Could you check a few things on this model? Use its own coordinates, in mm. Round coordinates to 2 decimals unless told otherwise and drop trailing zeros. Loops run counter-clockwise (first coordinate to the right, second up) from the corner with the lowest first, then second, coordinate; pieces in that order, holes last.
from build123d import *

# Parameters (mm, degrees)
SKETCH_1_W           = 250
SKETCH_1_H           = 140
EXTRUDE_1_DEPTH      = 4
SKETCH_2_R           = 1.55
CUT_EXTRUDE_1_DEPTH  = 4
SKETCH_4_W           = 350
SKETCH_4_H           = 30
EXTRUDE_2_DEPTH      = 4
EXTRUDE_3_DEPTH      = 4
SKETCH_3_R           = 2.05
CUT_EXTRUDE_2_DEPTH  = 4
SKETCH_6_W           = 189.5
SKETCH_6_H           = 45
CUT_EXTRUDE_3_DEPTH  = 4
CUT_EXTRUDE_4_DEPTH  = 4
CUT_EXTRUDE_5_DEPTH  = 4
FILLET_1_R           = 10
CUT_EXTRUDE_6_DEPTH  = 4
CUT_EXTRUDE_7_DEPTH  = 4
FILLET_2_R           = 2
FILLET_3_R           = 10
FILLET_4_R           = 30
SKETCH_11_R          = 1.55
EXTRUDE_4_DEPTH      = 4
EXTRUDE_START        = -4
EXTRUDE_5_DEPTH      = 4
SKETCH_13_R          = 2.1
CUT_EXTRUDE_12_DEPTH = 4
FILLET_5_R           = 2


with BuildPart() as part:
    # 草图1 → 凸台-拉伸1 (new body)
    with BuildSketch(Plane.XY):
        Rectangle(SKETCH_1_W, SKETCH_1_H)
    extrude(amount=EXTRUDE_1_DEPTH)

    # 草图2 → 切除-拉伸1 (cut)
    with BuildSketch(Plane.XY.offset(4)):
        with Locations((-108.75, 65)):
            Circle(SKETCH_2_R)
        with Locations((-108.75, 38.2)):
            Circle(SKETCH_2_R)
        with Locations((108.75, 65)):
            Circle(SKETCH_2_R)
        with Locations((108.75, 38.2)):
            Circle(SKETCH_2_R)
    extrude(amount=-CUT_EXTRUDE_1_DEPTH, mode=Mode.SUBTRACT)

    # 草图4 → 凸台-拉伸2 (add)
    with BuildSketch(Plane.XY.offset(4)):
        with Locations((0, -55)):
            Rectangle(SKETCH_4_W, SKETCH_4_H)
    extrude(amount=-EXTRUDE_2_DEPTH)

    # 草图5 → 凸台-拉伸3 (add)
    with BuildSketch(Plane.XY.offset(4)):
        Polygon((-125, -40), (-125, 70), (-175, -40), align=None)
        Polygon((175, -40), (125, 70), (125, -40), align=None)
    extrude(amount=-EXTRUDE_3_DEPTH)

    # 草图3 → 切除-拉伸2 (cut)
    with BuildSketch(Plane.XY.offset(4)):
        with Locations((50, -56.4)):
            Circle(SKETCH_3_R)
        with Locations((0, -56.4)):
            Circle(SKETCH_3_R)
        with Locations((100, -56.4)):
            Circle(SKETCH_3_R)
        with Locations((150, -56.4)):
            Circle(SKETCH_3_R)
        with Locations((-50, -56.4)):
            Circle(SKETCH_3_R)
        with Locations((-100, -56.4)):
            Circle(SKETCH_3_R)
        with Locations((-150, -56.4)):
            Circle(SKETCH_3_R)
    extrude(amount=-CUT_EXTRUDE_2_DEPTH, mode=Mode.SUBTRACT)

    # 草图6 → 切除-拉伸3 (cut)
    with BuildSketch(Plane.XY.offset(4)):
        with Locations((0, 47.5)):
            Rectangle(SKETCH_6_W, SKETCH_6_H)
    extrude(amount=-CUT_EXTRUDE_3_DEPTH, mode=Mode.SUBTRACT)

    # 草图7 → 切除-拉伸4 (cut)
    with BuildSketch(Plane.XY.offset(4)):
        Polygon((-125, 70), (-125, 30), (-175, -40), align=None)
        Polygon((175, -40), (125, 70), (125, 30), align=None)
    extrude(amount=-CUT_EXTRUDE_4_DEPTH, mode=Mode.SUBTRACT)

    # 草图8 → 切除-拉伸5 (cut)
    with BuildSketch(Plane.XY.offset(4)):
        with BuildLine():
            Line((-150, -63.9), (150, -63.9))
            ThreePointArc((150, -63.9), (156.178018616, -60.652303609), (157.005549561, -53.721889595))
            Line((157.005549561, -53.721889595), (125, 30))
            Line((125, 30), (228.155592589, 30))
            Line((228.155592589, 30), (175, -70))
            Line((175, -70), (-175, -70))
            Line((-175, -70), (-228.155592589, 30))
            Line((-228.155592589, 30), (-125, 30))
            Line((-125, 30), (-157.005549561, -53.721889595))
            ThreePointArc((-157.005549561, -53.721889595), (-156.178018616, -60.652303609), (-150, -63.9))
        make_face()
    extrude(amount=-CUT_EXTRUDE_5_DEPTH, mode=Mode.SUBTRACT)

    # 圆角1
    fillet_1_edges = [part.edges().sort_by_distance(p)[0] for p in [
        (94.75, 25, 2),
        (-94.75, 25, 2),
    ]]
    fillet(fillet_1_edges, radius=FILLET_1_R)

    # 草图9 → 切除-拉伸6 (cut)
    with BuildSketch(Plane.XY.offset(4)):
        Polygon((-57, -39.42450978), (-57, -46.4), (-4, -46.4), (-4, -22.251950414), align=None)
        Polygon((-57, -2.487306614), (-57, -28.912693386), (-16.221410479, -15.7), align=None)
        Polygon((-57, 15), (-57, 8.02450978), (-4, -9.148049586), (-4, 15), align=None)
        Polygon((4, 15), (4, -9.148049586), (57, 8.02450978), (57, 15), align=None)
        Polygon((16.221410479, -15.7), (57, -28.912693386), (57, -2.487306614), align=None)
        Polygon((4, -22.251950414), (4, -46.4), (57, -46.4), (57, -39.42450978), align=None)
        Polygon((63, -0.54324329), (63, -30.85675671), (94.75, -41.144091803), (94.75, 9.744091803), align=None)
        Polygon((-94.75, -41.144091803), (-63, -30.85675671), (-63, -0.54324329), (-94.75, 9.744091803), align=None)
    extrude(amount=-CUT_EXTRUDE_6_DEPTH, mode=Mode.SUBTRACT)

    # 草图10 → 切除-拉伸7 (cut)
    with BuildSketch(Plane.XY.offset(4)):
        Polygon((-100.75, 28.2), (-100.75, -46.4), (-145.641868809, -46.4), (-117.123472857, 28.2), align=None)
        Polygon((117.123472857, 28.2), (100.75, 28.2), (100.75, -46.4), (145.641868809, -46.4), align=None)
    extrude(amount=-CUT_EXTRUDE_7_DEPTH, mode=Mode.SUBTRACT)

    # 圆角2
    fillet_2_edges = [part.edges().sort_by_distance(p)[0] for p in [
        (-57, 15, 2),
        (-4, 15, 2),
        (-4, -9.148049586, 2),
        (-57, 8.02450978, 2),
        (-57, -2.487306614, 2),
        (-16.221410479, -15.7, 2),
        (-57, -28.912693386, 2),
        (57, -2.487306614, 2),
        (57, -28.912693386, 2),
        (16.221410479, -15.7, 2),
        (57, 15, 2),
        (57, 8.02450978, 2),
        (4, -9.148049586, 2),
        (4, 15, 2),
        (57, -39.42450978, 2),
        (57, -46.4, 2),
        (4, -46.4, 2),
        (4, -22.251950414, 2),
        (63, -0.54324329, 2),
        (94.75, 9.744091803, 2),
        (94.75, -41.144091803, 2),
        (63, -30.85675671, 2),
        (-63, -0.54324329, 2),
        (-63, -30.85675671, 2),
        (-94.75, -41.144091803, 2),
        (-94.75, 9.744091803, 2),
        (-57, -39.42450978, 2),
        (-4, -22.251950414, 2),
        (-4, -46.4, 2),
        (-57, -46.4, 2),
        (-100.75, -46.4, 2),
        (-145.641868809, -46.4, 2),
        (-117.123472857, 28.2, 2),
        (-100.75, 28.2, 2),
        (117.123472857, 28.2, 2),
        (145.641868809, -46.4, 2),
        (100.75, -46.4, 2),
        (100.75, 28.2, 2),
    ]]
    fillet(fillet_2_edges, radius=FILLET_2_R)

    # 圆角3
    fillet_3_edges = [part.edges().sort_by_distance(p)[0] for p in [
        (-94.75, 70, 2),
        (94.75, 70, 2),
        (-125, 70, 2),
        (125, 70, 2),
    ]]
    fillet(fillet_3_edges, radius=FILLET_3_R)

    # 圆角4
    fillet_4_edges = [part.edges().sort_by_distance(p)[0] for p in [
        (-125, 30, 2),
        (125, 30, 2),
    ]]
    fillet(fillet_4_edges, radius=FILLET_4_R)

    # 草图11 → 凸台-拉伸4 (add)
    with BuildSketch(Plane.XY.offset(4)):
        with Locations((108.75, 38.2)):
            Circle(SKETCH_11_R)
        with Locations((108.75, 65)):
            Circle(SKETCH_11_R)
        with Locations((-108.75, 38.2)):
            Circle(SKETCH_11_R)
        with Locations((-108.75, 65)):
            Circle(SKETCH_11_R)
    extrude(amount=-EXTRUDE_4_DEPTH)

    # 草图14 → 凸台-拉伸5 (add)
    with BuildSketch(Plane.XY.offset(4).offset(EXTRUDE_START)):
        with BuildLine():
            Line((100.75, 11.688155127), (120.935438111, 18.228450114))
            Line((120.935438111, 18.228450114), (117.61502802, 26.914162775))
            ThreePointArc((117.61502802, 26.914162775), (116.880829099, 27.847471631), (115.74688147, 28.2))
            Line((115.74688147, 28.2), (102.75, 28.2))
            ThreePointArc((102.75, 28.2), (101.335786438, 27.614213562), (100.75, 26.2))
            Line((100.75, 26.2), (100.75, 11.688155127))
        make_face()
        with BuildLine():
            Line((-100.75, 26.2), (-100.75, 11.688155127))
            Line((-100.75, 11.688155127), (-120.935438111, 18.228450114))
            Line((-120.935438111, 18.228450114), (-117.61502802, 26.914162775))
            ThreePointArc((-117.61502802, 26.914162775), (-116.880829099, 27.847471631), (-115.74688147, 28.2))
            Line((-115.74688147, 28.2), (-102.75, 28.2))
            ThreePointArc((-102.75, 28.2), (-101.335786438, 27.614213562), (-100.75, 26.2))
        make_face()
    extrude(amount=EXTRUDE_5_DEPTH)

    # 草图13 → 切除-拉伸12 (cut)
    with BuildSketch(Plane.XY.offset(4)):
        with Locations((112, 35.1)):
            Circle(SKETCH_13_R)
        with Locations((112, 64.1)):
            Circle(SKETCH_13_R)
        with Locations(Location((-112, 64.1, 0), (0, 0, 180))):
            Circle(SKETCH_13_R)
        with Locations(Location((-112, 35.1, 0), (0, 0, 180))):
            Circle(SKETCH_13_R)
    extrude(amount=-CUT_EXTRUDE_12_DEPTH, mode=Mode.SUBTRACT)

    # 圆角5
    fillet_5_edges = [part.edges().sort_by_distance(p)[0] for p in [
        (120.935438111, 18.228450114, 2),
        (100.75, 11.688155127, 2),
        (-120.935438111, 18.228450114, 2),
        (-100.75, 11.688155127, 2),
    ]]
    fillet(fillet_5_edges, radius=FILLET_5_R)


solid = part.part
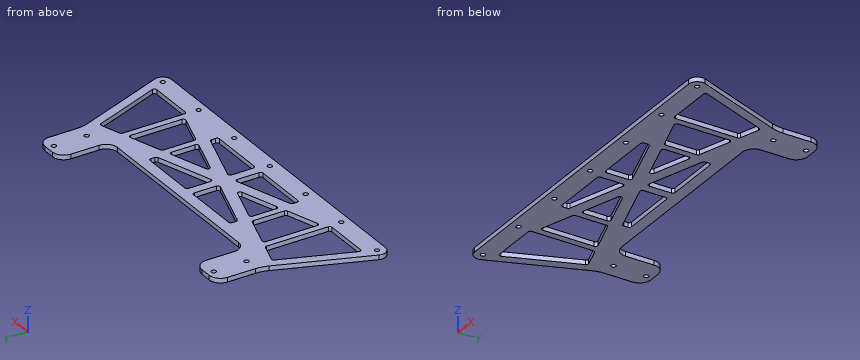
Item 1: If we section it at A-A, the plane x = 131.5: Please give me the cut outline in (y, z), then the cut area to 3 significant figures.
Results list:
outline: (-63.9, 0) - (-46.4, 0) - (-46.4, 4) - (-63.9, 4) - close; (-9.41, 0) - (13, 0) - (13, 4) - (-9.41, 4) - close
area: 160 mm2
Item 2: If we section it at C-C, the plane x = 33.5: Please give me the cut outline in (y, z), then the cut area to 3 significant figures.
Results list:
outline: (-63.9, 0) - (-46.4, 0) - (-46.4, 4) - (-63.9, 4) - close; (-31.81, 0) - (-21.3, 0) - (-21.3, 4) - (-31.81, 4) - close; (-10.1, 0) - (0.41, 0) - (0.41, 4) - (-10.1, 4) - close; (15, 0) - (25, 0) - (25, 4) - (15, 4) - close
area: 194 mm2
Item 3: Will these pins go through, and if not, where does the flat tip stop? pin 1 (2 mm diameter, centred on y = 45.5, z = 2, fed in from -X); pin 2 (1.5 mm diameter, centred on y = -27, z = 1.5, fed in from -X); pin 3 (1.8 mm diameter, centred on y = -42.5, z = 2.5, fed in from -X).
Results list:
pin 1: stops at x = -125
pin 2: stops at x = -147.08
pin 3: stops at x = -153.06
Item 4: If we section it at B-B, the plane y = 3.5: Please give me the cut outline in (x, z), then the cut area to 3 significant figures.
Results list:
outline: (-135.13, 0) - (-126.57, 0) - (-126.57, 4) - (-135.13, 4) - close; (-100.75, 0) - (-94.75, 0) - (-94.75, 4) - (-100.75, 4) - close; (-75.48, 0) - (-43.04, 0) - (-43.04, 4) - (-75.48, 4) - close; (-4, 0) - (4, 0) - (4, 4) - (-4, 4) - close; (43.04, 0) - (75.48, 0) - (75.48, 4) - (43.04, 4) - close; (94.75, 0) - (100.75, 0) - (100.75, 4) - (94.75, 4) - close; (126.57, 0) - (135.13, 0) - (135.13, 4) - (126.57, 4) - close
area: 408 mm2
Item 5: If we section it at D-D, the plane z = 3.3: Count the separate pieces of the cut face and the enclosed holes in it, then the cut area to 3 significant figures.
Results list:
separate pieces: 1
enclosed holes: 21
area: 17,100 mm2
Item 6: If I drill on line 1 along Y through (x, z) = (-112, 1.5); line 2 along Y through (x, z) = (-111.5, 2.75); line 3 along Y through (x, z) = (-59.5, 3.25), over which ranges is the centre line in solid material (lowest first)?
Results list:
line 1: y = -63.9 to -46.4, 15.33 to 33, 37.2 to 62, 66.2 to 70
line 2: y = -63.9 to -46.4, 15.17 to 33.06, 37.14 to 62.06, 66.14 to 70
line 3: y = -63.9 to 25
